```python
from build123d import *

# Parameters (mm, degrees)
F0_W     = 100
F0_H     = 200
F1_DEPTH = 100
F2_R     = 15
F3_DEPTH = 100
F5_DEPTH = 100


with BuildPart() as f1:
    # F0 (on Top) → F1 (new body)
    with BuildSketch(Plane.XY):
        Rectangle(F0_W, F0_H)
    extrude(amount=F1_DEPTH)

    # F2 (on face) → F3 (cut)
    with BuildSketch(Plane.XY.offset(100)):
        with Locations((18.2735839133, 40.5311594063)):
            Circle(F2_R)
    extrude(amount=-F3_DEPTH, mode=Mode.SUBTRACT)

    # F4 (on face) → F5 (cut)
    with BuildSketch(Plane.XY.offset(100)):
        with BuildLine():
            Line((33.9623928101, 100), (4.5817479461, 100))
            ThreePointArc((4.5817479461, 100), (19.2720703781, 88.0322313309), (33.9623928101, 100))
        make_face()
        with BuildLine():
            ThreePointArc((33.9623928101, 100), (34.1944501561, 101.5082294411), (34.2720703781, 103.0322313309))
            ThreePointArc((34.2720703781, 103.0322313309), (17.7480684883, 117.9546111089), (4.5817479461, 100))
            Line((4.5817479461, 100), (33.9623928101, 100))
        make_face()
    extrude(amount=-F5_DEPTH, mode=Mode.SUBTRACT)


solid = f1.part
```
Can you work these out from the model? Positions are in its coordinate system, mm. Round coordinates to 2 decimals unless told otherwise and drop trailing zeros. Loops run counter-clockwise (first coordinate to the right, second up) from the corner with the lowest first, then second, coordinate; pieces in that order, holes last. Notation, with made-up numbers: (36.5, 33.5) -> (54.5, 33.5) arc R21 cw to (54.5, 50.5) -> close; hole circle Ø9 at (-14, 57). An arc over 180 degrees is marked (long way). One line per item, written item: value. Start each with the question number.
1. If we section it at C-C, the plane y = 36.5: Write out the boundary of the cut face in (x, z).
2. If we mould it in two halves opening along Y, with no side actions, what happens to faces 1 (the flat face through (-1, 1, 100)), 2 (the cylindrical face through (16.3, 55.4, 50.7)), 3 (the flat face through (-1, -100, 49))? For each: pulls with the +Y half, pulls with the -Y half, needs draft (parallel to the pull), parting line crosses it, or undercut.
3. If we section it at B-B, the plane x = 8: Write out the boundary of the cut face in (y, z), then the cut area to 3 significant figures.
4. If I drill on probe 1 along Y at (x, z) = (9.5, 65.5); probe 2 along X at (y, z) = (43.5, 47.5); probe 3 along X at (y, z) = (32, 36), over which ranges is the centre line in solid material (lowest first)?
5. If we section it at A-A, the plane z = 92.5: Write out the boundary of the cut face in (x, y).
Calculated:
1. outline: (-50, 0) -> (3.83, 0) -> (3.83, 100) -> (-50, 100) -> close; (32.72, 0) -> (50, 0) -> (50, 100) -> (32.72, 100) -> close
2. face 1: needs draft
2. face 2: undercut
2. face 3: pulls with the -Y half
3. outline: (-100, 0) -> (29.6, 0) -> (29.6, 100) -> (-100, 100) -> close; (51.46, 0) -> (93.14, 0) -> (93.14, 100) -> (51.46, 100) -> close
3. area: 17,100 mm²
4. probe 1: y = -100 to 28.36, 52.7 to 91.65
4. probe 2: x = -50 to 3.57, 32.98 to 50
4. probe 3: x = -50 to 5.94, 30.61 to 50
5. outline: (-50, -100) -> (50, -100) -> (50, 100) -> (33.96, 100) arc R15 cw to (4.58, 100) -> (-50, 100) -> close; hole circle Ø30 at (18.27, 40.53)
